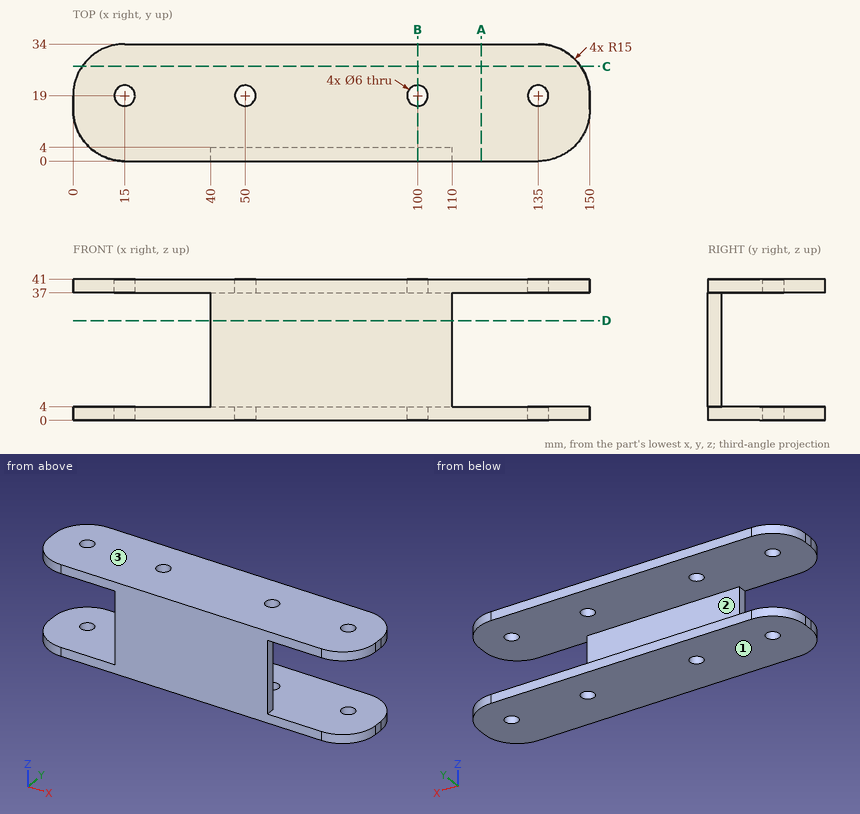
Geometry check sheet. Reference: drawing and pictorial views, mm from the part's lowest x, y, z. Give positions to 0.01 mm unless a question says otherwise; leave off trailing zeros. Order: outer loops, then holes, each group sorted by start corner. A loop starts at its lowest first (then second) coordinate and runs counter-clockwise, first axis right, second up. Notation, with made-up numbers: M -9,-21 L 46,-21 A11 cw 46,-7 Z; hole C -3,-6.5 d7. An arc over 180 degrees is marked long. Answer in a Markdown table with one row per item. Add a question column.
Q1. Sectioned sample at A-A, the plane x = 118.5. Record the boundary of the cut face in (y, z), and give its area (3 significant figures).
Q2. Gauge pin test, flat ends, axial feed: pin 1 Ø2 at (y, z) = (3, 25) entering from -X; pin 2 Ø5.5 at (x, y) = (100, 19) entering from +Z; pin 3 Ø1.5 at (x, z) = (54, 5) entering from +Y; pin 4 Ø4.5 at (y, z) = (2.5, 16.5) entering from +X. Record the tip position at first contact, or that the pin passes through.
Q3. Thickness scan on L1, parallel to Z at x = 15.5, y = 15; L2, parallel to Y at x = 135, z = 1.9; L3, parallel to Y at x = 80.5, z = 29. Record the ranges inside material, lowest first.
Q4. Sectioned sample at B-B, the plane x = 100. Record the boundary of the cut face in (y, z), and give its area (3 significant figures).
Q5. Release check for a two-part mould opening along Z. For the marked faces 1, 2 and 3 record: released by +Z, released by -Z, zero draft, split by the parting line, or undercut.
Q6. Sectioned sample at D-D, the plane z = 29. Record the boundary of the cut face in (x, y).
Q7. Sectioned sample at C-C, the plane y = 27.5. Record the boundary of the cut face in (x, z).
Verdict:
| question | item | result |
|---|---|---|
| 1 | outline | M 0,0 L 34,0 L 34,4 L 0,4 Z; M 0,37 L 34,37 L 34,41 L 0,41 Z |
| 1 | area | 272 mm² |
| 2 | pin 1 | x = 40 |
| 2 | pin 2 | through |
| 2 | pin 3 | y = 4 |
| 2 | pin 4 | x = 110 |
| 3 | L1 | 0 to 4, 37 to 41 |
| 3 | L2 | 0 to 16, 22 to 34 |
| 3 | L3 | 0 to 4 |
| 4 | outline | M 0,0 L 16,0 L 16,4 L 4,4 L 4,37 L 16,37 L 16,41 L 0,41 Z; M 22,0 L 34,0 L 34,4 L 22,4 Z; M 22,37 L 34,37 L 34,41 L 22,41 Z |
| 4 | area | 356 mm² |
| 5 | face 1 | released by -Z |
| 5 | face 2 | undercut |
| 5 | face 3 | released by +Z |
| 6 | outline | M 40,0 L 110,0 L 110,4 L 40,4 Z |
| 7 | outline | M 2.64,0 L 147.36,0 L 147.36,4 L 2.64,4 Z; M 2.64,37 L 147.36,37 L 147.36,41 L 2.64,41 Z |
